Part print with two shaded views. Sizes in mm from the minimum x, y, z corner. A direction names the side the tool comes from. Round coordinates to 2 decimals unless told otherwise and drop trailing zeros. Loops run counter-clockwise (first coordinate to the right, second up) from the corner with the lowest first, then second, coordinate; pieces in that order, holes last. Notation, with made-up numbers: (-5.75, 70.25) - (3.25, 70.25) arc R26 ccw to (3.25, 94.25) - close; hole circle Ø3 at (31.5, -36). An arc over 180 degrees is marked (long way). Write each question's results on one line, items separated by ' | '. Start each with the question number.
(1) Tool access for the marked faces 4 and 5: list every direction of +Z, -Z, +X, -X, +Y, -Y with a clear straight run to the whole face (end or side of a thin tool).
(2) Mould opens along Y. For the marked faces 1, 2 and 3 say: released by +Y, released by -Y, zero draft, split by the parting line, or undercut.
(3) Cut at C-C, the plane z = 6. List the corners of the cut face in (x, y) (1 decimal).
(4) Cut at A-A, the plane x = 26. List the corners of the cut face in (y, z) (1 decimal).
(5) Drill centre lines: L1, parallel to X at y = 21.5, z = 4.25 (1 decimal); L2, parallel to Y at x = 48, z = 4.5 (1 decimal); L3, parallel to Z at x = 25, y = 32.5. Where is each one in solid material? Low to high.
(6) Flat gauge pins, fed straight in: P1, Ø8, axis at x = 39, y = 6, coming from the -Z side; P2, Ø1.5, axis at x = 22, y = 18.5, coming from the +Z side. Where does each tip first touch, or does it go through?
(7) Cut at B-B, the plane y = 28.5. List the corners of the cut face in (x, z) (1 decimal).
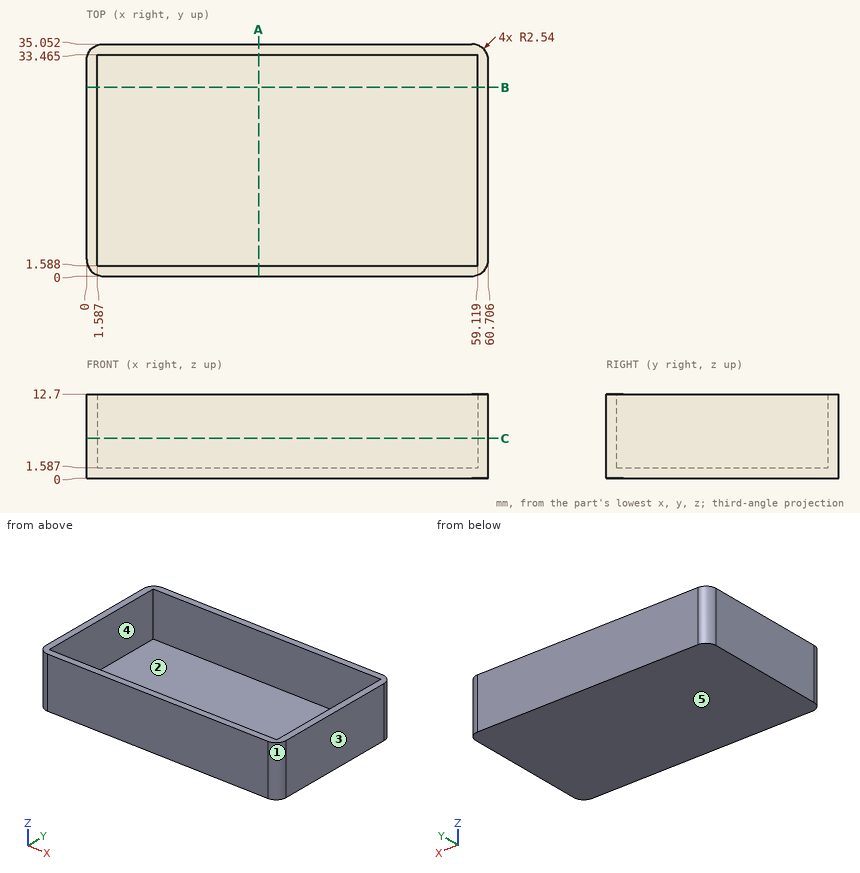
A:
1) face 4: +Z | face 5: -Z, +X, -X, +Y, -Y
2) face 1: released by -Y | face 2: undercut | face 3: zero draft
3) outline: (0, 2.5) arc R2.5 ccw to (2.5, 0) - (58.2, 0) arc R2.5 ccw to (60.7, 2.5) - (60.7, 32.5) arc R2.5 ccw to (58.2, 35.1) - (2.5, 35.1) arc R2.5 ccw to (0, 32.5) - close; hole (1.6, 1.6) - (59.1, 1.6) - (59.1, 33.5) - (1.6, 33.5) - close
4) outline: (0, 0) - (35.1, 0) - (35.1, 12.7) - (33.5, 12.7) - (33.5, 1.6) - (1.6, 1.6) - (1.6, 12.7) - (0, 12.7) - close
5) L1: 0 to 1.6, 59.1 to 60.7 | L2: 0 to 1.6, 33.5 to 35.1 | L3: 0 to 1.59
6) P1: z = 0 | P2: z = 1.59
7) outline: (0, 0) - (60.7, 0) - (60.7, 12.7) - (59.1, 12.7) - (59.1, 1.6) - (1.6, 1.6) - (1.6, 12.7) - (0, 12.7) - close
